Geometry: see drawing. Coordinates: mm, zero at the bounding-box minimum. A direction names the side the tool comes from. Round coordinates to 2 decimals unless told otherwise and drop trailing zeros. Write each loop counter-clockwise with the first axis right and the second up, starting at its lowest first coordinate (ties: lowest second). Pieces come first, ordered by that corner, then holes.
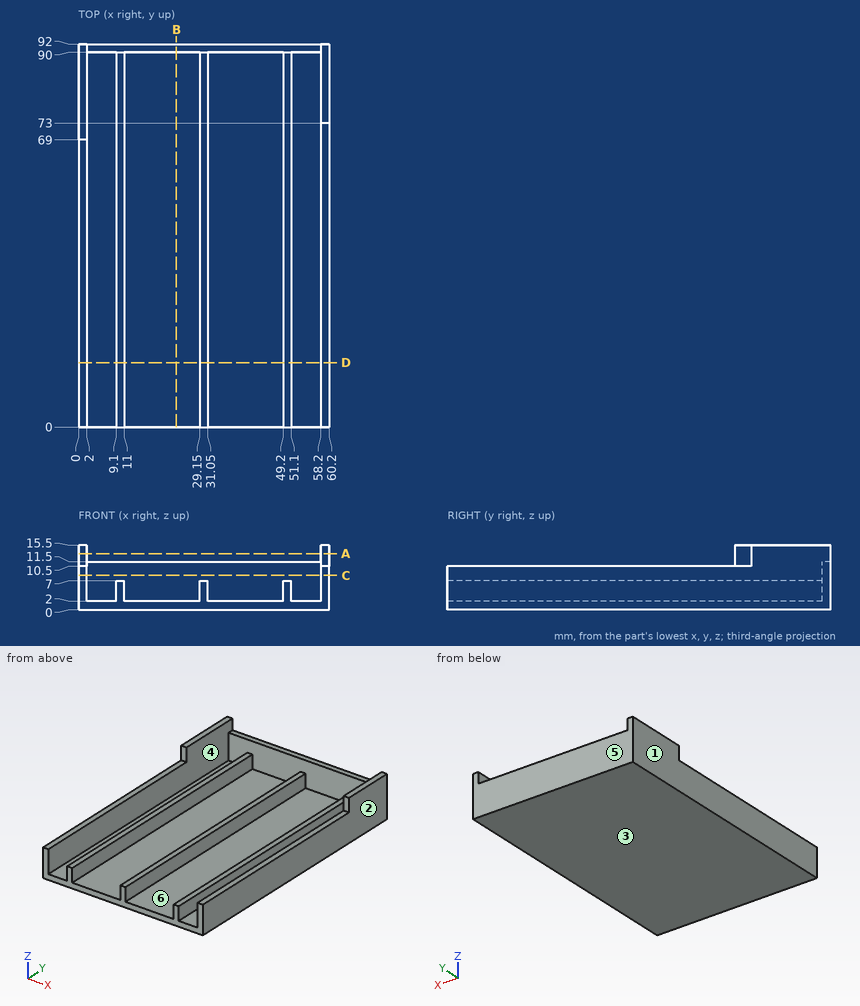
1) Pull-direction query (X, two-part tool) for the marked faces 1, 2, 3 and 4; classes: released by +X, released by -X, zero draft, split by the parting line, or undercut.
Taken from the geometry:
face 1: released by -X
face 2: released by +X
face 3: zero draft
face 4: undercut
2) Section query C-C on z = 8.25. Return the cut outline in (x, y), then the cut area to 3 significant figures.
Taken from the geometry:
outline: (0, 0) - (2, 0) - (2, 90) - (58.2, 90) - (58.2, 0) - (60.2, 0) - (60.2, 92) - (0, 92) - close
area: 480 mm2
3) Reachability of the marked faces 5 and 6 from +Z, -Z, +X, -X, +Y, -Y: full face, straight path, thin tool, end or side. Return the list, or none.
Taken from the geometry:
face 5: +Z, -Z, +X, -X, +Y
face 6: +Z, -Y
4) Section query B-B on x = 23.5. Return the cut outline in (y, z), then the cut area to 3 significant figures.
Taken from the geometry:
outline: (0, 0) - (92, 0) - (92, 11.5) - (90, 11.5) - (90, 2) - (0, 2) - close
area: 203 mm2
5) Material intervals for line 1 (X direction, y = 34, z = 4); line 2 (X direction, y = 78.5, z = 14.5); line 3 (Z direction, x = 37, y = 76), sorted ascending.
Taken from the geometry:
line 1: x = 0 to 2, 9.1 to 11, 29.15 to 31.05, 49.2 to 51.1, 58.2 to 60.2
line 2: x = 0 to 2, 58.2 to 60.2
line 3: z = 0 to 2
6) Section query D-D on y = 15.5. Return the cut outline in (x, z).
Taken from the geometry:
outline: (0, 0) - (60.2, 0) - (60.2, 10.5) - (58.2, 10.5) - (58.2, 2) - (51.1, 2) - (51.1, 7) - (49.2, 7) - (49.2, 2) - (31.05, 2) - (31.05, 7) - (29.15, 7) - (29.15, 2) - (11, 2) - (11, 7) - (9.1, 7) - (9.1, 2) - (2, 2) - (2, 10.5) - (0, 10.5) - close
7) Contact query for flat-ended pins moving along their axis: P1, Ø2, axis at x = 50, y = 26, coming from the +Z side; P2, Ø2, axis at x = 56.5, y = 60.5, coming from the +Z side; P3, Ø4, axis at y = 56.5, z = 5.5, coming from the -X side; P4, Ø0.6, axis at x = 59, z = 14, coming from the -Y side. Output: stop coordinate, or through.
Taken from the geometry:
P1: stops at z = 7
P2: stops at z = 2
P3: stops at x = 0
P4: stops at y = 73
8) Section query A-A on z = 13.5. Return the cut outline in (x, y), then the cut area to 3 significant figures.
Taken from the geometry:
outline: (0, 69) - (2, 69) - (2, 92) - (0, 92) - close; (58.2, 73) - (60.2, 73) - (60.2, 92) - (58.2, 92) - close
area: 84.0 mm2
